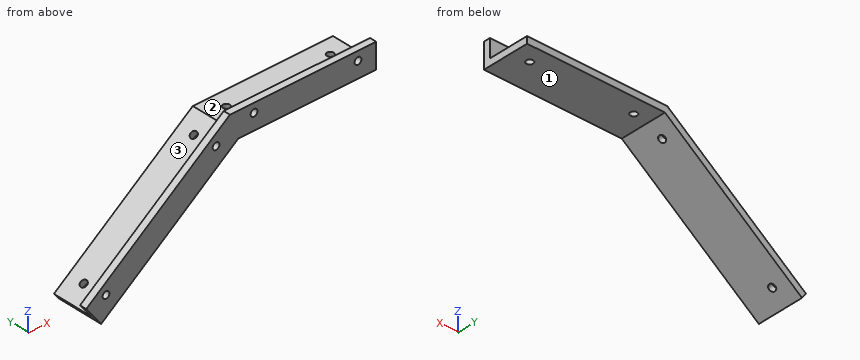
```python
from build123d import *

# Parameters (mm, degrees)
SALIENTE_EXTRUIR4_DEPTH      = 3
SALIENTE_EXTRUIR6_DEPTH      = 18
SALIENTE_EXTRUIR6_DEPTH_BACK = 3
CROQUIS5_R                   = 1.5
CORTAR_EXTRUIR2_DEPTH        = 3
CROQUIS6_R                   = 1.5
CORTAR_EXTRUIR3_DEPTH        = 3
CROQUIS7_R                   = 1.5
CORTAR_EXTRUIR5_DEPTH        = 3
CROQUIS8_R                   = 1.5
CORTAR_EXTRUIR6_DEPTH        = 3
CROQUIS9_R                   = 1.5
CORTAR_EXTRUIR7_DEPTH        = 3
CROQUIS10_R                  = 1.5
SALIENTE_EXTRUIR7_DEPTH      = 3


with BuildPart() as part:
    # Croquis1 → Saliente-Extruir4 (new body)
    with BuildSketch(Plane(origin=(0, 0, 0), x_dir=(1, 0, 0), z_dir=(0, 1, 0))):
        Polygon((0, 0), (-62, 0), (-123.446373684, 46.404128707), (-128.267581862, 40.020089883), (-64.681421115, -8), (0, -8), align=None)
    extrude(amount=SALIENTE_EXTRUIR4_DEPTH)

    # Croquis4 → Saliente-Extruir6 (add, two sides: drawn at the far end of the back side and taken through both)
    with BuildSketch(Plane(origin=(0, 3, 0), x_dir=(1, 0, 0), z_dir=(0, 1, 0)).offset(-SALIENTE_EXTRUIR6_DEPTH_BACK)):
        Polygon((-123.446373684, 46.404128707), (-121.638420618, 48.798143266), (-60.994467082, 3), (0, 3), (0, 0), (-62, 0), align=None)
    extrude(amount=SALIENTE_EXTRUIR6_DEPTH + SALIENTE_EXTRUIR6_DEPTH_BACK)

    # Croquis5 → Cortar-Extruir2 (cut)
    with BuildSketch(Plane(origin=(0, 3, 0), x_dir=(1, 0, 0), z_dir=(0, 1, 0))):
        with Locations(Location((-4, -4, 0), (0, 0, 270))):
            Circle(CROQUIS5_R)
        with Locations(Location((-58, -4, 0), (0, 0, 270))):
            Circle(CROQUIS5_R)
    extrude(amount=-CORTAR_EXTRUIR2_DEPTH, mode=Mode.SUBTRACT)

    # Croquis6 → Cortar-Extruir3 (cut)
    with BuildSketch(Plane(origin=(0, 3, 0), x_dir=(1, 0, 0), z_dir=(0, 1, 0))):
        with Locations(Location((-122.664958361, 40.801505206, 0), (0, 0, 270))):
            Circle(CROQUIS6_R)
        with Locations(Location((-67.602623501, -0.781415324, 0), (0, 0, 270))):
            Circle(CROQUIS6_R)
    extrude(amount=-CORTAR_EXTRUIR3_DEPTH, mode=Mode.SUBTRACT)

    # Croquis7 → Cortar-Extruir5 (cut)
    with BuildSketch(Plane(origin=(-22.51767178, 0, 29.816943304), x_dir=(0.7980048530430802, 0, 0.6026510221676322), z_dir=(-0.6026510221676322, 0, 0.7980048530430802))):
        with Locations((-118.476300889, 13.5)):
            Circle(CROQUIS7_R)
        with Locations((-57.476300889, 13.5)):
            Circle(CROQUIS7_R)
    extrude(amount=-CORTAR_EXTRUIR5_DEPTH, mode=Mode.SUBTRACT)

    # Croquis8 → Cortar-Extruir6 (cut)
    with BuildSketch(Plane.XY):
        with Locations((-54, 13.5)):
            Circle(CROQUIS8_R)
        with Locations((-8, 13.5)):
            Circle(CROQUIS8_R)
    extrude(amount=-CORTAR_EXTRUIR6_DEPTH, mode=Mode.SUBTRACT)

    # Croquis9 → Cortar-Extruir7 (cut)
    with BuildSketch(Plane(origin=(0, 3, 0), x_dir=(1, 0, 0), z_dir=(0, 1, 0))):
        with Locations(Location((-119.472938949, 38.390901117, 0), (0, 0, 270))):
            Circle(CROQUIS9_R)
        with Locations(Location((-70.794642913, 1.629188765, 0), (0, 0, 270))):
            Circle(CROQUIS9_R)
        with Locations(Location((-54, -4, 0), (0, 0, 270))):
            Circle(CROQUIS9_R)
        with Locations(Location((-8, -4, 0), (0, 0, 270))):
            Circle(CROQUIS9_R)
    extrude(amount=-CORTAR_EXTRUIR7_DEPTH, mode=Mode.SUBTRACT)

    # Croquis10 → Saliente-Extruir7 (add)
    with BuildSketch(Plane(origin=(0, 3, 0), x_dir=(1, 0, 0), z_dir=(0, 1, 0))):
        with Locations((-58, -4)):
            Circle(CROQUIS10_R)
        with Locations((-4, -4)):
            Circle(CROQUIS10_R)
        with Locations((-67.602623501, -0.781415324)):
            Circle(CROQUIS10_R)
        with Locations((-122.664958361, 40.801505206)):
            Circle(CROQUIS10_R)
    extrude(amount=-SALIENTE_EXTRUIR7_DEPTH)


solid = part.part
```
Build history of the part. All positions in model axes, mm. Face numbers are marked on the shaded views. A direction names the side the tool comes from. Round coordinates to 2 decimals unless told otherwise and drop trailing zeros. Order: outer loops, then holes, each group sorted by start corner. A loop starts at its lowest first (then second) coordinate and runs counter-clockwise, first axis right, second up. Notation, with made-up numbers: (55.5, 85.5) -> (95.5, 85.5) arc R18 cw to (95.5, 91.5) -> close; hole circle Ø6 at (0.5, -30). An arc over 180 degrees is marked (long way). Answer in a Markdown table with one row per item.
1) Band-saw the part on C-C on x = -33.5. Give the cut face in (y, z), and give its area (3 significant figures).
Values:
| item | result |
|---|---|
| outline | (0, -3) -> (21, -3) -> (21, 0) -> (3, 0) -> (3, 8) -> (0, 8) -> close |
| area | 87.0 mm2 |
2) Pin check, flat tips, straight feed: P1, Ø8, axis at x = -103.5, y = 4, coming from the +Z side; P2, Ø2, axis at x = -27.5, y = 17, coming from the -Z side; P3, Ø1.8, axis at x = -119.47, z = -38.39, coming from the -Y side; P4, Ø6, axis at x = -68, y = 16, coming from the +Z side. Stop position of each tip, or through.
Values:
| item | result |
|---|---|
| P1 | z = -18.39 |
| P2 | z = -3 |
| P3 | through |
| P4 | z = -2.27 |
3) Band-saw the part on D-D on y = 6.25. Give the cut face in (x, z).
Values:
| item | result |
|---|---|
| outline | (-123.45, -46.4) -> (-121.64, -48.8) -> (-60.99, -3) -> (0, -3) -> (0, 0) -> (-62, 0) -> close |
4) Band-saw the part on B-B on z = 4. Give the cut face in (x, y).
Values:
| item | result |
|---|---|
| outline | (-69.98, 0) -> (-55.5, 0) -> (-55.5, 3) -> (-69.98, 3) -> close; (-52.5, 0) -> (-9.5, 0) -> (-9.5, 3) -> (-52.5, 3) -> close; (-6.5, 0) -> (0, 0) -> (0, 3) -> (-6.5, 3) -> close |
5) Band-saw the part on A-A on x = -54. Give the cut face in (y, z), and give its area (3 significant figures).
Values:
| item | result |
|---|---|
| outline | (0, -3) -> (12, -3) -> (12, 0) -> (3, 0) -> (3, 2.5) -> (0, 2.5) -> close; (0, 5.5) -> (3, 5.5) -> (3, 8) -> (0, 8) -> close; (15, -3) -> (21, -3) -> (21, 0) -> (15, 0) -> close |
| area | 69.0 mm2 |
6) Wall check: L1, parallel to X at y = 2.25, z = 4; L2, parallel to Z at x = -38.5, y = 3.75; L3, parallel to Y at x = -117.5, z = -33.5. Give the ranges that are in metal, low to high.
Values:
| item | result |
|---|---|
| L1 | -69.98 to -55.5, -52.5 to -9.5, -6.5 to 0 |
| L2 | -3 to 0 |
| L3 | 0 to 3 |
7) Which spindle directions (+Z, -Z, +X, -X, +Y, -Y) get a long thin tool onto all of the face, cutting with end or side? Do the marked faces 1, 2 and 3. Say none if no direction does.
Values:
| item | result |
|---|---|
| face 1 | -Z, +X, +Y, -Y |
| face 2 | +Z, +X, -X, +Y |
| face 3 | +Z, -X, +Y |
